Can you work these out from the model? Positions are in its coordinate system, mm. A direction names the side the tool comes from. Round coordinates to 2 decimals unless told otherwise and drop trailing zeros. Write each loop counter-clockwise with the first axis right and the second up, starting at its lowest first coordinate (ties: lowest second). Pieces come first, ordered by that corner, then holes. Notation, with made-up numbers: M 42.5,-4 L 98.5,-4 A29 cw 98.5,32 Z; hole C 32,37.25 d3. An arc over 180 degrees is marked long. Answer as a JSON object with one key per item and string values. Group by question number.
1) I'm going to push flat-ended pins straight in: pin 1 Ø1.5 at (y, z) = (-14.5, 29) entering from +X; pin 2 Ø8 at (x, z) = (-50.34, 21.71) entering from +Y; pin 3 Ø1 at (y, z) = (-5, 23.5) entering from +X; pin 4 Ø1 at (x, y) = (-91.5, -12) entering from +Z. Where does each tip first touch, or does it pass through?
2) Suppose I cut it at A-A, the plane y = -8.5. Write out the boundary of the cut face in (x, z) (3 decimals).
3) Please list where these lines run through material, in increasing order: L1, parallel to X at y = -15.5, z = 25; L2, parallel to X at y = -1.75, z = 18; L3, parallel to X at y = -17, z = 22. Write a range as [from, to].
4) On a 3-axis mill with a long thin cutter (end or side, diameter ignored), from which of +Z, -Z, +X, -X, +Y, -Y can I reach the whole of each face in a straight line? I mean faces 3 (the flat face through (-75.7, -2.5, 11.1)), 4 (the flat face through (-97, 0, 15)). Say none if no direction works.
5) If we mould it in two halves opening along X, with no side actions, what happens to faces 1 (the flat face through (-97, -19.05, 22)), 2 (the cylindrical face through (-148.674, -6.887, 21.413))? For each: +X half, -X half, draft (parallel to the pull), parting line (faces both ways), or undercut.
6) Suppose I cut it at B-B, the plane x = -142. Write out the boundary of the cut face in (y, z).
7) Suppose I cut it at D-D, the plane x = -83. Write out the boundary of the cut face in (y, z), and give its area (3 significant figures).
8) Suppose I cut it at C-C, the plane y = -2.25. Write out the boundary of the cut face in (x, z) (3 decimals), and give its area (3 significant figures).
from build123d import *

# Parameters (mm, degrees)
F0_R     = 4.445
F1_DEPTH = 19.05
F3_DEPTH = 13.97
F4_R     = 5.08
F5_DEPTH = 5.08


with BuildPart() as f1:
    # F0 (on Front) → F1 (new body)
    with BuildSketch(Plane.XZ):
        with BuildLine():
            ThreePointArc((-124.9322268395, 28.7639294598), (-130.4980059639, 35.017678352), (-138.4710976488, 37.5705358593))
            ThreePointArc((-138.4710976488, 37.5705358593), (-155.0254015346, 22.0518028606), (-139.1540765762, 5.8352343242))
            Line((-139.1540765762, 5.8352343242), (-137.7946125004, 5.8935506507))
            ThreePointArc((-137.7946125004, 5.8935506507), (-130.1034423833, 8.6679321614), (-124.8131018813, 14.9019988847))
            Line((-124.8131018813, 14.9019988847), (-133.3336122029, 14.1704850261))
            ThreePointArc((-133.3336122029, 14.1704850261), (-148.6790765762, 21.7102343242), (-133.3336122029, 29.2499836224))
            Line((-133.3336122029, 29.2499836224), (-124.9322268395, 28.7639294598))
        make_face()
        with BuildLine():
            Line((-99.1008544222, 34.8894799677), (-99.1008544222, 35.8751666308))
            Line((-99.1008544222, 35.8751666308), (-138.4710976488, 37.5705358593))
            ThreePointArc((-138.4710976488, 37.5705358593), (-130.4980059639, 35.017678352), (-124.9322268395, 28.7639294598))
            Line((-124.9322268395, 28.7639294598), (-110.4319389367, 27.9250290893))
            ThreePointArc((-110.4319389367, 27.9250290893), (-105.7509869831, 33.0091720577), (-99.1008544222, 34.8894799677))
        make_face()
        with BuildLine():
            Line((-137.7946125004, 5.8935506507), (-99.0179549294, 7.5569357044))
            Line((-99.0179549294, 7.5569357044), (-99.1008544222, 9.4894799677))
            ThreePointArc((-99.1008544222, 9.4894799677), (-105.6044119808, 11.2810548255), (-110.273070294, 16.1503084588))
            Line((-110.273070294, 16.1503084588), (-124.8131018813, 14.9019988847))
            ThreePointArc((-124.8131018813, 14.9019988847), (-130.1034423833, 8.6679321614), (-137.7946125004, 5.8935506507))
        make_face()
        with BuildLine():
            ThreePointArc((-99.1008544222, 9.4894799677), (-96.8524942518, 9.6900849205), (-94.6751627721, 10.2855624017))
            ThreePointArc((-94.6751627721, 10.2855624017), (-88.6726167006, 14.9409036921), (-86.4008544222, 22.1894799677))
            Line((-86.4008544222, 22.1894799677), (-94.0208544222, 22.1894799677))
            ThreePointArc((-94.0208544222, 22.1894799677), (-95.5087519738, 18.5973775193), (-99.1008544222, 17.1094799677))
            Line((-99.1008544222, 17.1094799677), (-110.273070294, 16.1503084588))
            ThreePointArc((-110.273070294, 16.1503084588), (-105.6044119808, 11.2810548255), (-99.1008544222, 9.4894799677))
        make_face()
        with BuildLine():
            ThreePointArc((-86.4008544222, 22.1894799677), (-88.0348602906, 28.4211550137), (-92.5164093638, 33.0492720132))
            ThreePointArc((-92.5164093638, 33.0492720132), (-95.6824746143, 34.4207791419), (-99.1008544222, 34.8894799677))
            ThreePointArc((-99.1008544222, 34.8894799677), (-105.7509869831, 33.0091720577), (-110.4319389367, 27.9250290893))
            Line((-110.4319389367, 27.9250290893), (-99.1008544222, 27.2694799677))
            ThreePointArc((-99.1008544222, 27.2694799677), (-95.5087519738, 25.7815824161), (-94.0208544222, 22.1894799677))
            Line((-94.0208544222, 22.1894799677), (-86.4008544222, 22.1894799677))
        make_face()
        with BuildLine():
            Line((-99.0179549294, 7.5569357044), (-87.6442336226, 8.0448291746))
            Line((-87.6442336226, 8.0448291746), (-87.7530907655, 10.5824954495))
            Line((-87.7530907655, 10.5824954495), (-94.6751627721, 10.2855624017))
            ThreePointArc((-94.6751627721, 10.2855624017), (-96.8524942518, 9.6900849205), (-99.1008544222, 9.4894799677))
            Line((-99.1008544222, 9.4894799677), (-99.0179549294, 7.5569357044))
        make_face()
        with BuildLine():
            Line((-86.5101311345, 32.7906284679), (-86.4008544222, 35.3282767099))
            Line((-86.4008544222, 35.3282767099), (-99.1008544222, 35.8751666308))
            Line((-99.1008544222, 35.8751666308), (-99.1008544222, 34.8894799677))
            ThreePointArc((-99.1008544222, 34.8894799677), (-95.6824746143, 34.4207791419), (-92.5164093638, 33.0492720132))
            Line((-92.5164093638, 33.0492720132), (-86.5101311345, 32.7906284679))
        make_face()
        with BuildLine():
            ThreePointArc((-57.3392350777, 31.5344655517), (-54.0123637648, 33.2013955962), (-50.3357569569, 33.7752343242))
            Line((-50.3357569569, 33.7752343242), (-86.4008544222, 35.3282767099))
            Line((-86.4008544222, 35.3282767099), (-86.5101311345, 32.7906284679))
            Line((-86.5101311345, 32.7906284679), (-57.3392350777, 31.5344655517))
        make_face()
        with BuildLine():
            Line((-87.6442336226, 8.0448291746), (-50.3357569569, 9.6452343242))
            ThreePointArc((-50.3357569569, 9.6452343242), (-54.0132473827, 10.2193558039), (-57.3407458906, 11.8870802972))
            Line((-57.3407458906, 11.8870802972), (-87.7530907655, 10.5824954495))
            Line((-87.7530907655, 10.5824954495), (-87.6442336226, 8.0448291746))
        make_face()
        with BuildLine():
            ThreePointArc((-50.3357569569, 9.6452343242), (-41.8045136419, 13.1789910092), (-38.2707569569, 21.7102343242))
            ThreePointArc((-38.2707569569, 21.7102343242), (-41.8045136419, 30.2414776392), (-50.3357569569, 33.7752343242))
            ThreePointArc((-50.3357569569, 33.7752343242), (-54.0123637648, 33.2013955962), (-57.3392350777, 31.5344655517))
            ThreePointArc((-57.3392350777, 31.5344655517), (-62.4007569212, 21.7111620791), (-57.3407458906, 11.8870802972))
            ThreePointArc((-57.3407458906, 11.8870802972), (-54.0132473827, 10.2193558039), (-50.3357569569, 9.6452343242))
        make_face()
        with Locations((-50.3357569569, 21.7102343242)):
            Circle(F0_R, mode=Mode.SUBTRACT)
    extrude(amount=F1_DEPTH)

    # F2 (on face) → F3 (join)
    with BuildSketch(Plane.XZ.offset(19.05)):
        with BuildLine():
            ThreePointArc((-86.4008544222, 22.1894799677), (-88.6726167006, 14.9409036921), (-94.6751627721, 10.2855624017))
            Line((-94.6751627721, 10.2855624017), (-57.3407458906, 11.8870802972))
            ThreePointArc((-57.3407458906, 11.8870802972), (-62.4007569212, 21.7111620791), (-57.3392350777, 31.5344655517))
            Line((-57.3392350777, 31.5344655517), (-92.5164093638, 33.0492720132))
            ThreePointArc((-92.5164093638, 33.0492720132), (-88.0348602906, 28.4211550137), (-86.4008544222, 22.1894799677))
        make_face()
        with BuildLine():
            Line((-57.3407458906, 11.8870802972), (-94.6751627721, 10.2855624017))
            ThreePointArc((-94.6751627721, 10.2855624017), (-103.5704974557, 10.301995324), (-110.273070294, 16.1503084588))
            Line((-110.273070294, 16.1503084588), (-133.3336122029, 14.1704850261))
            ThreePointArc((-133.3336122029, 14.1704850261), (-148.6790765762, 21.7102343242), (-133.3336122029, 29.2499836224))
            Line((-133.3336122029, 29.2499836224), (-110.4319389367, 27.9250290893))
            ThreePointArc((-110.4319389367, 27.9250290893), (-102.5932909524, 34.3998397938), (-92.5164093638, 33.0492720132))
            Line((-92.5164093638, 33.0492720132), (-57.3392350777, 31.5344655517))
            ThreePointArc((-57.3392350777, 31.5344655517), (-54.0123637648, 33.2013955962), (-50.3357569569, 33.7752343242))
            Line((-50.3357569569, 33.7752343242), (-138.4710976488, 37.5705358593))
            ThreePointArc((-138.4710976488, 37.5705358593), (-155.0254015346, 22.0518028606), (-139.1540765762, 5.8352343242))
            Line((-139.1540765762, 5.8352343242), (-50.3357569569, 9.6452343242))
            ThreePointArc((-50.3357569569, 9.6452343242), (-54.0132473827, 10.2193558039), (-57.3407458906, 11.8870802972))
        make_face()
    extrude(amount=-F3_DEPTH)

    # F4 (on face) → F5 (join)
    with BuildSketch(Plane.XZ.offset(19.05)):
        with BuildLine():
            ThreePointArc((-133.3336122029, 29.2499836224), (-148.6790765762, 21.7102343242), (-133.3336122029, 14.1704850261))
            ThreePointArc((-133.3336122029, 14.1704850261), (-130.6052302168, 17.5098949424), (-129.6290765762, 21.7102343242))
            ThreePointArc((-129.6290765762, 21.7102343242), (-130.6052302168, 25.910573706), (-133.3336122029, 29.2499836224))
        make_face()
        with Locations((-139.1540765762, 21.7102343242)):
            Circle(F4_R, mode=Mode.SUBTRACT)
        with BuildLine():
            ThreePointArc((-129.6290765762, 21.7102343242), (-130.6052302168, 17.5098949424), (-133.3336122029, 14.1704850261))
            Line((-133.3336122029, 14.1704850261), (-99.1008544222, 17.1094799677))
            ThreePointArc((-99.1008544222, 17.1094799677), (-104.1808544222, 22.1894799677), (-99.1008544222, 27.2694799677))
            Line((-99.1008544222, 27.2694799677), (-133.3336122029, 29.2499836224))
            ThreePointArc((-133.3336122029, 29.2499836224), (-130.6052302168, 25.910573706), (-129.6290765762, 21.7102343242))
        make_face()
        with BuildLine():
            ThreePointArc((-99.1008544222, 27.2694799677), (-104.1808544222, 22.1894799677), (-99.1008544222, 17.1094799677))
            ThreePointArc((-99.1008544222, 17.1094799677), (-95.5087519738, 18.5973775193), (-94.0208544222, 22.1894799677))
            ThreePointArc((-94.0208544222, 22.1894799677), (-95.5087519738, 25.7815824161), (-99.1008544222, 27.2694799677))
        make_face()
    extrude(amount=-F5_DEPTH)


solid = f1.part
Results:
{
 "1": {"pin 1": "x = -40.2", "pin 2": "through", "pin 3": "x = -38.34", "pin 4": "z = 35.57"},
 "2": {"outline": "M -139.154,5.835 L -50.336,9.645 A12.065 ccw -50.336,33.775 L -138.471,37.571 A15.875 ccw long Z; hole M -133.334,14.17 L -99.101,17.109 A5.08 ccw -99.101,27.269 L -133.334,29.25 A9.525 ccw long Z; hole C -50.336,21.71 d8.89"},
 "3": {"L1": "[-154.68, -143.02], [-135.28, -53.32], [-47.35, -38.73]", "L2": "[-154.59, -147.93], [-96.23, -87.11], [-61.82, -52.78], [-47.89, -38.86]", "L3": "[-155.03, -144.23], [-134.08, -54.77], [-45.9, -38.27]"},
 "4": {"face 3": "+Y", "face 4": "+Z, -Z, +X, -X, +Y"},
 "5": {"face 1": "draft", "face 2": "undercut"},
 "6": {"outline": "M -19.05,6.09 L 0,6.09 L 0,12.62 L -13.97,12.62 L -13.97,17.5 L -19.05,17.5 Z; M -19.05,25.92 L -13.97,25.92 L -13.97,30.8 L 0,30.8 L 0,37.33 L -19.05,37.33 Z"},
 "7": {"outline": "M -19.05,8.24 L 0,8.24 L 0,10.79 L -5.08,10.79 L -5.08,32.64 L 0,32.64 L 0,35.18 L -19.05,35.18 Z", "area": "402 mm^2"},
 "8": {"outline": "M -139.154,5.835 L -50.336,9.645 A12.065 ccw -50.336,33.775 L -138.471,37.571 A15.875 ccw long Z; hole M -133.334,14.17 L -99.101,17.109 A5.08 ccw -99.101,27.269 L -133.334,29.25 A9.525 ccw long Z; hole M -94.675,10.286 L -57.341,11.887 A12.065 cw -57.339,31.534 L -92.516,33.049 A12.7 cw Z; hole C -50.336,21.71 d8.89", "area": "1,740 mm^2"}
}
